```python
from build123d import *

# Parameters (mm, degrees)
SKETCH_2_W          = 10
SKETCH_2_H          = 10
SKETCH_2_W_2        = 8
SKETCH_2_H_2        = 8
EXTRUDE_1_DEPTH     = 31.3
CUT_EXTRUDE_1_REACH = 36.347
SKETCH_3_R          = 1.6
CUT_EXTRUDE_2_REACH = 36.347
SKETCH_4_R          = 1.6


with BuildPart() as part:
    # ｽｹｯﾁ2 → 押し出し-薄板1 (new body)
    with BuildSketch(Plane.XY):
        with Locations((5, 5)):
            Rectangle(SKETCH_2_W, SKETCH_2_H)
        with Locations((5, 5)):
            Rectangle(SKETCH_2_W_2, SKETCH_2_H_2, mode=Mode.SUBTRACT)
    extrude(amount=EXTRUDE_1_DEPTH)

    # ｶｯﾄ - 押し出し1: up to this face of the body (flat: up to its plane)
    cut_extrude_1_end = Plane(part.part.faces().sort_by_distance((5, 0, 15.65))[0])
    # ｽｹｯﾁ3 → ｶｯﾄ - 押し出し1 (cut, up to the picked face)
    with BuildSketch(Plane(origin=(0, 10, 0), x_dir=(1, 0, 0), z_dir=(0, 1, 0)), mode=Mode.PRIVATE) as cut_extrude_1_sk1:
        with Locations(Location((5, -23.15, 0), (0, 0, 270))):
            Circle(SKETCH_3_R)
    cut_extrude_1_tool1 = split(extrude(cut_extrude_1_sk1.sketch, amount=-CUT_EXTRUDE_1_REACH, mode=Mode.PRIVATE), bisect_by=cut_extrude_1_end, keep=Keep.BOTH, mode=Mode.PRIVATE)
    # ｽｹｯﾁ3 → ｶｯﾄ - 押し出し1 (cut, up to the picked face)
    with BuildSketch(Plane(origin=(0, 10, 0), x_dir=(1, 0, 0), z_dir=(0, 1, 0)), mode=Mode.PRIVATE) as cut_extrude_1_sk2:
        with Locations(Location((5, -8.15, 0), (0, 0, 270))):
            Circle(SKETCH_3_R)
    cut_extrude_1_tool2 = split(extrude(cut_extrude_1_sk2.sketch, amount=-CUT_EXTRUDE_1_REACH, mode=Mode.PRIVATE), bisect_by=cut_extrude_1_end, keep=Keep.BOTH, mode=Mode.PRIVATE)
    add(cut_extrude_1_tool1.solids().sort_by(Axis((5, 10, 23.15), (0, -1, 0)))[0], mode=Mode.SUBTRACT)
    add(cut_extrude_1_tool2.solids().sort_by(Axis((5, 10, 8.15), (0, -1, 0)))[0], mode=Mode.SUBTRACT)

    # ｶｯﾄ - 押し出し2: up to this face of the body (flat: up to its plane)
    cut_extrude_2_end = Plane(part.part.faces().sort_by_distance((0, 5, 15.65))[0])
    # ｽｹｯﾁ4 → ｶｯﾄ - 押し出し2 (cut, up to the picked face)
    with BuildSketch(Plane(origin=(10, 0, 0), x_dir=(0, 0, -1), z_dir=(1, 0, 0)), mode=Mode.PRIVATE) as cut_extrude_2_sk1:
        with Locations((-28.35, 5)):
            Circle(SKETCH_4_R)
    cut_extrude_2_tool1 = split(extrude(cut_extrude_2_sk1.sketch, amount=-CUT_EXTRUDE_2_REACH, mode=Mode.PRIVATE), bisect_by=cut_extrude_2_end, keep=Keep.BOTH, mode=Mode.PRIVATE)
    # ｽｹｯﾁ4 → ｶｯﾄ - 押し出し2 (cut, up to the picked face)
    with BuildSketch(Plane(origin=(10, 0, 0), x_dir=(0, 0, -1), z_dir=(1, 0, 0)), mode=Mode.PRIVATE) as cut_extrude_2_sk2:
        with Locations(Location((-2.95, 5, 0), (0, 0, 180))):
            Circle(SKETCH_4_R)
    cut_extrude_2_tool2 = split(extrude(cut_extrude_2_sk2.sketch, amount=-CUT_EXTRUDE_2_REACH, mode=Mode.PRIVATE), bisect_by=cut_extrude_2_end, keep=Keep.BOTH, mode=Mode.PRIVATE)
    add(cut_extrude_2_tool1.solids().sort_by(Axis((10, 5, 28.35), (-1, 0, 0)))[0], mode=Mode.SUBTRACT)
    add(cut_extrude_2_tool2.solids().sort_by(Axis((10, 5, 2.95), (-1, 0, 0)))[0], mode=Mode.SUBTRACT)


solid = part.part
```
Verification items for the finished model (mm, model axes). A direction names the side the tool comes from. Coordinates: 2 decimals unless noted, no trailing zeros. Loops run counter-clockwise (first coordinate to the right, second up) from the corner with the lowest first, then second, coordinate; pieces in that order, holes last. Notation, with made-up numbers: (-27, 60) - (12, 60) arc R5 ccw to (12, 66) - close; hole circle Ø1 at (79, -20.5). An arc over 180 degrees is marked (long way). Return JSON: item names as keys, results as strings.
1. Mould release check, pull along Y, two halves, no side actions. Record for faces 3 (the flat face through (5, 1, 15)), 4 (the flat face through (5, 10, 15)), 5 (the cylindrical face through (3.44, 0.51, 7.8)): +Y half, -Y half, draft (parallel to the pull), parting line (faces both ways), or undercut.
Established:
{"face 3": "undercut", "face 4": "+Y half", "face 5": "draft"}
2. Go/stop test with a flat-tipped pin: pin 1 (1.9 mm diameter, centred on y = 5, z = 28.35, fed in from +X). Record where the tip stops, or that it passes through.
Established:
{"pin 1": "passes through"}
3. Tool access check on faces 1 (the flat face through (1, 5, 15)), 2 (the flat face through (0, 5, 15)). Record the directions out of +Z, -Z, +X, -X, +Y, -Y that give a thin tool (end or side, any length) a straight path to the whole face; none if there is none.
Established:
{"face 1": "+Z, -Z", "face 2": "+Z, -Z, -X, +Y, -Y"}
4. Section check C-C, the plane z = 5.5. Record the boundary of the cut face in (x, y).
Established:
{"outline": "(0, 0) - (10, 0) - (10, 10) - (0, 10) - close; hole (1, 1) - (9, 1) - (9, 9) - (1, 9) - close"}
5. Section check A-A, the plane x = 5. Record the boundary of the cut face in (y, z), then the cut area to 3 significant figures.
Established:
{"outline": "(0, 0) - (1, 0) - (1, 6.55) - (0, 6.55) - close; (0, 9.75) - (1, 9.75) - (1, 21.55) - (0, 21.55) - close; (0, 24.75) - (1, 24.75) - (1, 31.3) - (0, 31.3) - close; (9, 0) - (10, 0) - (10, 6.55) - (9, 6.55) - close; (9, 9.75) - (10, 9.75) - (10, 21.55) - (9, 21.55) - close; (9, 24.75) - (10, 24.75) - (10, 31.3) - (9, 31.3) - close", "area": "49.8 mm2"}
6. Thickness scan on L1, parallel to X at y = 1.25, z = 7; L2, parallel to Y at x = 0.45, z = 2.95. Record the ranges inside material, lowest first.
Established:
{"L1": "x = 0 to 1, 9 to 10", "L2": "y = 0 to 3.4, 6.6 to 10"}
7. Section check B-B, the plane y = 1.5. Record the boundary of the cut face in (x, z).
Established:
{"outline": "(0, 0) - (1, 0) - (1, 31.3) - (0, 31.3) - close; (9, 0) - (10, 0) - (10, 31.3) - (9, 31.3) - close"}
